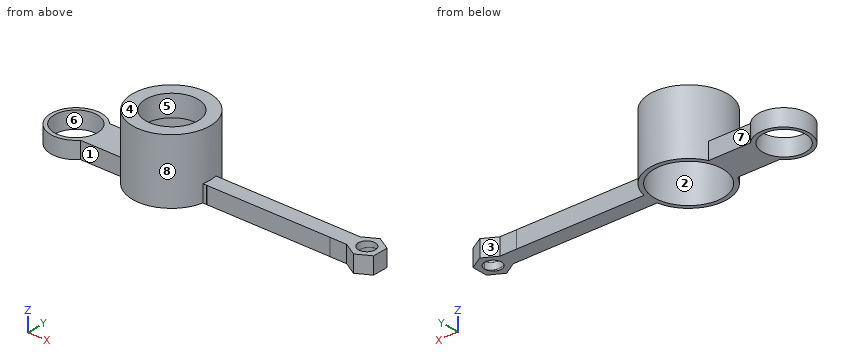
```python
from build123d import *

# Parameters (mm, degrees)
BOSS_EXTRUDE1_DEPTH     = 10
CUT_EXTRUDE1_DEPTH      = 10
CUT_EXTRUDE1_DEPTH_BACK = 10
SKETCH2_R               = 5
CUT_SWEEP1_PITCH        = 4
CUT_SWEEP1_HEIGHT       = 10
CUT_SWEEP1_RADIUS       = 5
EXTRUDE_THIN2_DEPTH     = 10
BODY_MOVE_COPY1_ANGLE   = 2
SKETCH10_W              = 73.109037791
SKETCH10_H              = 9.197874715
BOSS_EXTRUDE2_DEPTH     = 10
SKETCH14_W              = 2.398597497
SKETCH14_H              = 9.211550244
BOSS_EXTRUDE7_DEPTH     = 10
SKETCH14_3_R            = 22.86
BOSS_EXTRUDE8_DEPTH     = 38.1
CUT_EXTRUDE2_DEPTH      = 25.4
CUT_EXTRUDE2_DEPTH_BACK = 38.1
SKETCH15_R              = 20.32
CUT_EXTRUDE3_DEPTH      = 38.1
CUT_EXTRUDE3_DEPTH_BACK = 38.1
SKETCH16_R              = 15.4
SKETCH17_W              = 25.201116709
SKETCH17_H              = 20.14431591
BOSS_EXTRUDE9_DEPTH     = 10
SKETCH19_R              = 15
BOSS_EXTRUDE10_DEPTH    = 10
CUT_EXTRUDE4_DEPTH      = 10
CUT_EXTRUDE4_DEPTH_BACK = 10
SKETCH20_R              = 12.7


with BuildPart() as part:
    # Sketch1 → Boss-Extrude1 (new body)
    with BuildSketch(Plane.XY):
        Polygon((-8.167579482, -4.315550803), (-0.346413115, -9.231106721), (7.821166368, -4.915555918), (8.167579482, 4.315550803), (0.346413115, 9.231106721), (-7.821166368, 4.915555918), align=None)
    extrude(amount=BOSS_EXTRUDE1_DEPTH)

    # Sketch2 → Cut-Extrude1 (cut, two sides: drawn at the far end of the back side and taken through both)
    with BuildSketch(Plane.XY.offset(-CUT_EXTRUDE1_DEPTH_BACK)):
        Circle(SKETCH2_R)
    extrude(amount=CUT_EXTRUDE1_DEPTH + CUT_EXTRUDE1_DEPTH_BACK, mode=Mode.SUBTRACT)

    # Cut-Sweep1: sweep along a helix
    with BuildLine() as cut_sweep1_path:
        Helix(CUT_SWEEP1_PITCH, CUT_SWEEP1_HEIGHT, CUT_SWEEP1_RADIUS, center=(0, 0, 0), direction=(0, 0, 1), lefthand=True)
    # Sketch4 → Cut-Sweep1 (sweep, cut)
    with BuildSketch(Plane.XY):
        Polygon((5.337109255, 0), (4.831445373, 0.291945178), (4.831445373, -0.291945178), align=None)
    sweep(path=cut_sweep1_path.line, is_frenet=True, mode=Mode.SUBTRACT)

    # Sketch6 → Extrude-Thin2 (add)
    with BuildSketch(Plane.XY):
        Polygon((-7.821166368, 4.915555918), (-8.167579482, -4.315550803), (-18.160545639, -3.940547606), (-17.814132524, 5.290559115), align=None)
    extrude(amount=EXTRUDE_THIN2_DEPTH)


with BuildPart() as part_1:
    # Body-Move/Copy1: moved
    add(part.part.rotate(Axis((-4.996483078, 0, 0), (0, 0, 1)), BODY_MOVE_COPY1_ANGLE))

    # Sketch10 → Boss-Extrude2 (add)
    with BuildSketch(Plane.XY):
        with Locations((-54.545481105, 0.241069377)):
            Rectangle(SKETCH10_W, SKETCH10_H)
    extrude(amount=BOSS_EXTRUDE2_DEPTH)

    # Sketch14 → Boss-Extrude7 (add)
    with BuildSketch(Plane.XY):
        with Locations((-92.299298749, 0.234231612)):
            Rectangle(SKETCH14_W, SKETCH14_H)
    extrude(amount=BOSS_EXTRUDE7_DEPTH)

    # Sketch14<3> → Boss-Extrude8 (add)
    with BuildSketch(Plane.XY):
        with Locations(Location((-115.84035067, 0, 0), (0, 0, 12.223392191))):
            Circle(SKETCH14_3_R)
    extrude(amount=BOSS_EXTRUDE8_DEPTH)

    # Sketch15 → Cut-Extrude2 (cut, two sides: drawn at the far end of the back side and taken through both)
    with BuildSketch(Plane.XY.offset(-CUT_EXTRUDE2_DEPTH_BACK)):
        with Locations((-115.84035067, 0)):
            Circle(SKETCH15_R)
    extrude(amount=CUT_EXTRUDE2_DEPTH + CUT_EXTRUDE2_DEPTH_BACK, mode=Mode.SUBTRACT)

    # Sketch16 → Cut-Extrude3 (cut, two sides: drawn at the far end of the back side and taken through both)
    with BuildSketch(Plane.XY.offset(-CUT_EXTRUDE3_DEPTH_BACK)):
        with Locations(Location((-115.534237584, 0, 0), (0, 0, 180))):
            Circle(SKETCH16_R)
    extrude(amount=CUT_EXTRUDE3_DEPTH + CUT_EXTRUDE3_DEPTH_BACK, mode=Mode.SUBTRACT)

    # Sketch17 → Boss-Extrude9 (add)
    with BuildSketch(Plane.XY):
        with Locations((-148.962391284, 0)):
            Rectangle(SKETCH17_W, SKETCH17_H)
    extrude(amount=BOSS_EXTRUDE9_DEPTH)

    # Sketch19 → Boss-Extrude10 (add)
    with BuildSketch(Plane.XY):
        with Locations((-172.255338782, 0)):
            Circle(SKETCH19_R)
    extrude(amount=BOSS_EXTRUDE10_DEPTH)

    # Sketch20 → Cut-Extrude4 (cut, two sides: drawn at the far end of the back side and taken through both)
    with BuildSketch(Plane.XY.offset(-CUT_EXTRUDE4_DEPTH_BACK)):
        with Locations((-172.49769937, 0)):
            Circle(SKETCH20_R)
    extrude(amount=CUT_EXTRUDE4_DEPTH + CUT_EXTRUDE4_DEPTH_BACK, mode=Mode.SUBTRACT)


solid = part_1.part
```
Model file for the job. Use its own axes, mm. Face numbers are marked on the shaded views. A direction names the side the tool comes from. Round coordinates to 2 decimals unless told otherwise and drop trailing zeros. Write each loop counter-clockwise with the first axis right and the second up, starting at its lowest first coordinate (ties: lowest second). Pieces come first, ordered by that corner, then holes. Notation, with made-up numbers: M -3.75,37.25 L 54.25,37.25 A24 cw 54.25,57.25 Z; hole C -30.75,-28.5 d1. An arc over 180 degrees is marked long. Put each result on its own line as item: value.
Item 1: Cut at C-C (y = 17.5). List the corners of the cut face in (x, z), and give its area (3 significant figures).
Responses:
outline: M -130.55,0 L -126.17,0 L -126.17,25.4 L -105.51,25.4 L -105.51,0 L -101.13,0 L -101.13,38.1 L -130.55,38.1 Z
area: 596 mm²
Item 2: Cut at B-B (z = 13). List the corners of the cut face in (x, y), and give its area (3 significant figures).
Responses:
outline: C -115.84,0 d45.72; hole C -115.84,0 d40.64
area: 345 mm²
Item 3: Flat gauge pins, fed straight in: P1, Ø8, axis at x = -31, z = 12.5, coming from the +Y side; P2, Ø8, axis at x = -157.5, z = 5, coming from the +Y side; P3, Ø3, axis at y = -4, z = 22, coming from the +X side. Where does each tip first touch, or does it go through?
Responses:
P1: y = 4.84
P2: y = 10.46
P3: x = -93.12
Item 4: Probe L1, parallel to X at y = 0, z = 3.75; L2, parallel to X at y = -13, z = 2; L3, parallel to Z at x = -99, y = -10.5. List the from-to ranges inside material, lowest first. Write a range as from..to.
Responses:
L1: -187.26..-185.2, -159.8..-136.16, -95.52..-5, 4.99..8
L2: -179.74..-164.77, -134.64..-131.46, -100.22..-97.04
L3: 25.4..38.1
Item 5: Cut at D-D (x = -134.5). List the corners of the cut face in (y, z), and give its area (3 significant figures).
Responses:
outline: M -13.21,0 L -8.04,0 L -8.04,25.4 L 8.04,25.4 L 8.04,0 L 13.21,0 L 13.21,38.1 L -13.21,38.1 Z
area: 598 mm²
Item 6: Tool access for the marked faces 1, 2, 3 and 4: list every direction of +Z, -Z, +X, -X, +Y, -Y with a clear straight run to the whole face (end or side of a thin tool).
Responses:
face 1: +Z, -Z, -Y
face 2: -Z
face 3: +Z, -Z, +Y
face 4: +Z, +X, -X, +Y, -Y
Item 7: Cut at A-A (x = -113.5). List the corners of the cut face in (y, z).
Responses:
outline: M -22.74,0 L -20.18,0 L -20.18,25.4 L -15.27,25.4 L -15.27,38.1 L -22.74,38.1 Z; M 15.27,25.4 L 20.18,25.4 L 20.18,0 L 22.74,0 L 22.74,38.1 L 15.27,38.1 Z
Item 8: Mould opens along Y. For the marked faces 5, 6, 7 and 8 say: +Y half, -Y half, draft (parallel to the pull), parting line (faces both ways), or undercut.
Responses:
face 5: undercut
face 6: undercut
face 7: +Y half
face 8: parting line
